Model file for the job. Use its own axes, mm. A direction names the side the tool comes from. Round coordinates to 2 decimals unless told otherwise and drop trailing zeros. Loops run counter-clockwise (first coordinate to the right, second up) from the corner with the lowest first, then second, coordinate; pieces in that order, holes last. Notation, with made-up numbers: M 17.25,-12 L 44.25,-12 A32 cw 44.25,15 Z; hole C 77,37.5 d4. An arc over 180 degrees is marked long. Use a Markdown table: item, result. Add a question column.
Q1. Cut at B-B (x = 0). Give the cut face in (y, z).
Q2. Cut at C-C (x = 13.5). Give the cut face in (y, z).
Q3. Probe line 1 (Y direction, x = 0, z = 1.8); line 2 (Y direction, x = -20.5, z = -2.65); line 3 (X direction, y = 3.5, z = 2.5). List the from-to ranges inside material, lowest first. Write a range as from..to.
Q4. Pin check, flat tips, straight feed: pin 1 (0.6 mm diameter, centred on y = -7, z = 0.5, fed in from +X); pin 2 (1.8 mm diameter, centred on x = 14.5, z = -0.5, fed in from -Y); pin 3 (2 mm diameter, centred on y = 10.5, z = 0, fed in from +X). Stop position of each tip, or through.
Q5. Cut at A-A (z = -2.1). Give the cut face in (x, y).
Q6. Cut at D-D (y = 24.5). Give the cut face in (x, z).
Q7. Tool access for faces 1 (the face through (7.69, -3.37, 0.04)), 2 (the face through (-1.82, -8.63, 0.04)), 3 (the face through (-4.97, 5, 0.04)): list every direction of +Z, -Z, +X, -X, +Y, -Y with a clear straight run to the whole face (end or side of a thin tool).
Q8. Mould opens along X. For faces 4 (the face through (1.048, -8.773, 0.042)), 5 (the face through (12, 13.923, 0)), 6 (the face through (-4.478, -7.957, 0.042)) say: +X half, -X half, draft (parallel to the pull), parting line (faces both ways), or undercut.
from build123d import *

# Parameters (mm, degrees)
SKETCH_1_R      = 2.05
EXTRUDE_1_DEPTH = 3


with BuildPart() as part:
    # 스케치1 → 보스-돌출1 (new, symmetric)
    with BuildSketch(Plane.XY):
        with BuildLine():
            Line((-3.714453644, -0.659762387), (-2.378622648, -5.81789167))
            Line((-2.378622648, -5.81789167), (-4.775045742, -6.743825318))
            Line((-4.775045742, -6.743825318), (-4.17347403, -9.205553558))
            Line((-4.17347403, -9.205553558), (0.595403586, -8.040184518))
            Line((0.595403586, -8.040184518), (1.5135427, -9.526878273))
            Line((1.5135427, -9.526878273), (8.699439255, -7.770863118))
            Line((8.699439255, -7.770863118), (8.699439255, -6.62630488))
            ThreePointArc((8.699439255, -6.62630488), (7.437294697, -6.763917269), (6.342454802, -6.121055183))
            Line((6.342454802, -6.121055183), (5.976753085, -3.963411438))
            Line((5.976753085, -3.963411438), (9.448395839, -2.762750085))
            Line((9.448395839, -2.762750085), (9.643145165, -1.456614425))
            Line((9.643145165, -1.456614425), (5.558763062, -0.851575902))
            Line((5.558763062, -0.851575902), (5.384598497, 0.445037535))
            ThreePointArc((5.384598497, 0.445037535), (6.001978603, 2.68132709), (7.290465917, 4.61056259))
            ThreePointArc((7.290465917, 4.61056259), (9.349741981, 6.480399593), (11.856878684, 7.685046382))
            Line((11.856878684, 7.685046382), (18.984206684, 7.685046382))
            Line((18.984206684, 7.685046382), (18.984206684, 11.608441399))
            ThreePointArc((18.984206684, 11.608441399), (18.747143867, 13.056663145), (17.562507461, 13.922793382))
            Line((17.562507461, 13.922793382), (5.368815069, 13.922793382))
            ThreePointArc((5.368815069, 13.922793382), (-0.689207057, 15.930226431), (-3.717586974, 21.547906968))
            ThreePointArc((-3.717586974, 21.547906968), (-13.434946181, 25.571091327), (-23.817349178, 27.25001668))
            ThreePointArc((-23.817349178, 27.25001668), (-24.977134733, 24.378166735), (-22.105284788, 23.21838118))
            ThreePointArc((-22.105284788, 23.21838118), (-13.06126812, 21.129967821), (-5.487273706, 15.764306963))
            ThreePointArc((-5.487273706, 15.764306963), (-5.434873097, 12.848146862), (-8.232673416, 12.024102607))
            ThreePointArc((-8.232673416, 12.024102607), (-9.017409998, 10.65199102), (-8.87513846, 9.077741828))
            ThreePointArc((-8.87513846, 9.077741828), (-4.931237162, 4.931648988), (-3.714453644, -0.659762387))
        make_face()
        Circle(SKETCH_1_R, mode=Mode.SUBTRACT)
    extrude(amount=EXTRUDE_1_DEPTH, both=True)


solid = part.part
Checked values:
| question | item | result |
|---|---|---|
| 1 | outline | M -8.19,-3 L -2.05,-3 L -2.05,3 L -8.19,3 Z; M 2.05,-3 L 15.41,-3 L 15.41,3 L 2.05,3 Z |
| 2 | outline | M 7.69,-3 L 13.92,-3 L 13.92,3 L 7.69,3 Z |
| 3 | line 1 | y = -8.19..-2.05, 2.05..15.41 |
| 3 | line 2 | y = 23.11..26.98 |
| 3 | line 3 | x = -4.3..6.44 |
| 4 | pin 1 | stops at x = 8.7 |
| 4 | pin 2 | stops at y = 7.69 |
| 4 | pin 3 | stops at x = 18.98 |
| 5 | outline | M -23.82,27.25 A2.19 ccw -22.11,23.22 A23.99 cw -5.49,15.76 A2.41 cw -8.23,12.02 A2.63 ccw -8.88,9.08 A10.61 cw -3.71,-0.66 L -2.38,-5.82 L -4.78,-6.74 L -4.17,-9.21 L 0.6,-8.04 L 1.51,-9.53 L 8.7,-7.77 L 8.7,-6.63 A2.02 cw 6.34,-6.12 L 5.98,-3.96 L 9.45,-2.76 L 9.64,-1.46 L 5.56,-0.85 L 5.38,0.45 A7.29 cw 7.29,4.61 A9.65 cw 11.86,7.69 L 18.98,7.69 L 18.98,11.61 A1.94 ccw 17.56,13.92 L 5.37,13.92 A8.64 cw -3.72,21.55 A45.39 ccw Z; hole C 0,0 d4.1 |
| 6 | outline | M -25.02,-3 L -10.14,-3 L -10.14,3 L -25.02,3 Z |
| 7 | face 1 | +Z, -Z, +X |
| 7 | face 2 | +Z, -Z, -Y |
| 7 | face 3 | +Z, -Z, -X |
| 8 | face 4 | undercut |
| 8 | face 5 | draft |
| 8 | face 6 | -X half |
